Part model, mm, in its own coordinate system. A direction names the side the tool comes from. Give positions to 0.01 mm unless a question says otherwise; leave off trailing zeros. Order: outer loops, then holes, each group sorted by start corner. A loop starts at its lowest first (then second) coordinate and runs counter-clockwise, first axis right, second up. Notation, with made-up numbers: (48.5, 12) - (67.5, 12) arc R37 cw to (67.5, 51) - close; hole circle Ø6 at (65, 52.25). An arc over 180 degrees is marked (long way). One line per item, written item: value.
```python
from build123d import *

# Parameters (mm, degrees)
SKETCH1_R           = 15.875
BOSS_EXTRUDE1_DEPTH = 3.175
SKETCH2_R           = 14.2875
BOSS_EXTRUDE2_DEPTH = 6.35
CUT_EXTRUDE1_DEPTH  = 10.525


with BuildPart() as part:
    # Sketch1 → Boss-Extrude1 (new body)
    with BuildSketch(Plane(origin=(0, 0, 0), x_dir=(0, 0, -1), z_dir=(1, 0, 0))):
        Circle(SKETCH1_R)
    extrude(amount=BOSS_EXTRUDE1_DEPTH)

    # Sketch2 → Boss-Extrude2 (add)
    with BuildSketch(Plane(origin=(3.175, 0, 0), x_dir=(0, 0, -1), z_dir=(1, 0, 0))):
        Circle(SKETCH2_R)
    extrude(amount=BOSS_EXTRUDE2_DEPTH)

    # Sketch3 → Cut-Extrude1 (cut, through all)
    with BuildSketch(Plane(origin=(9.525, 0, 0), x_dir=(0, 0, -1), z_dir=(1, 0, 0))):
        Polygon((7.332348419, 0), (3.666174209, 6.35), (-3.666174209, 6.35), (-7.332348419, 0), (-3.666174209, -6.35), (3.666174209, -6.35), align=None)
    extrude(amount=-CUT_EXTRUDE1_DEPTH, mode=Mode.SUBTRACT)


solid = part.part
```
1) Drill centre lines: line 1 along Y through (x, z) = (7.5, -5); line 2 along Y through (x, z) = (2.5, -4.5); line 3 along Z through (x, y) = (2, -4). Where is each one in solid material? Low to high. Write a range as from..to.
Outcome:
line 1: y = -13.38..-4.04, 4.04..13.38
line 2: y = -15.22..-4.91, 4.91..15.22
line 3: z = -15.36..-5.02, 5.02..15.36
2) Cut at C-C, the plane y = 8.5. Give the cut face in (x, z) (3 decimals), then the cut area to 3 significant figures.
Outcome:
outline: (0, -13.408) - (3.175, -13.408) - (3.175, -11.484) - (9.525, -11.484) - (9.525, 11.484) - (3.175, 11.484) - (3.175, 13.408) - (0, 13.408) - close
area: 231 mm^2
3) Which spindle directions (+Z, -Z, +X, -X, +Y, -Y) get a long thin tool onto all of the face, cutting with end or side? Do faces 1 (the flat face through (3.175, 8.31, 11.83)), 2 (the flat face through (4.829, 3.131, -5.525)), 3 (the flat face through (9.525, 7, 0)). Say none if no direction does.
Outcome:
face 1: +X
face 2: +X, -X
face 3: +Z, -Z, +X, +Y, -Y
4) Pin check, flat tips, straight feed: pin 1 (1 mm diameter, centred on x = 4.5, z = -11, fed in from -Y); pin 2 (3 mm diameter, centred on x = 7, z = -1.5, fed in from -Y); pin 3 (1 mm diameter, centred on x = 8, y = -11, fed in from -Z). Stop position of each tip, or through.
Outcome:
pin 1: stops at y = -9.69
pin 2: stops at y = -14.29
pin 3: stops at z = -9.69
5) Mould opens along Z. For faces 4 (the flat face through (4.829, 3.219, 5.474)), 5 (the cylindrical face through (6.306, 0.628, 14.274)), 6 (the flat face through (0, -7, 0)) say: released by +Z, released by -Z, zero draft, split by the parting line, or undercut.
Outcome:
face 4: undercut
face 5: split by the parting line
face 6: zero draft
6) Cut at D-D, the plane x = 1.5. Give the cut face in (y, z) (3 decimals), then the cut area to 3 significant figures.
Outcome:
outline: circle Ø31.75 at (0, 0); hole (-6.35, -3.666) - (0, -7.332) - (6.35, -3.666) - (6.35, 3.666) - (0, 7.332) - (-6.35, 3.666) - close
area: 652 mm^2
